Drawing for the job (mm, zero at the part's lowest x, y, z). Round coordinates to 2 decimals unless told otherwise and drop trailing zeros. Write each loop counter-clockwise with the first axis right and the second up, starting at its lowest first coordinate (ties: lowest second). Pieces come first, ordered by that corner, then holes. Notation, with made-up numbers: (-23.75, 77.25) - (3.25, 77.25) arc R21 cw to (3.25, 106.25) - close; hole circle Ø5 at (-19.75, 24). An arc over 180 degrees is marked (long way). One line per question, with ' | ' between items.
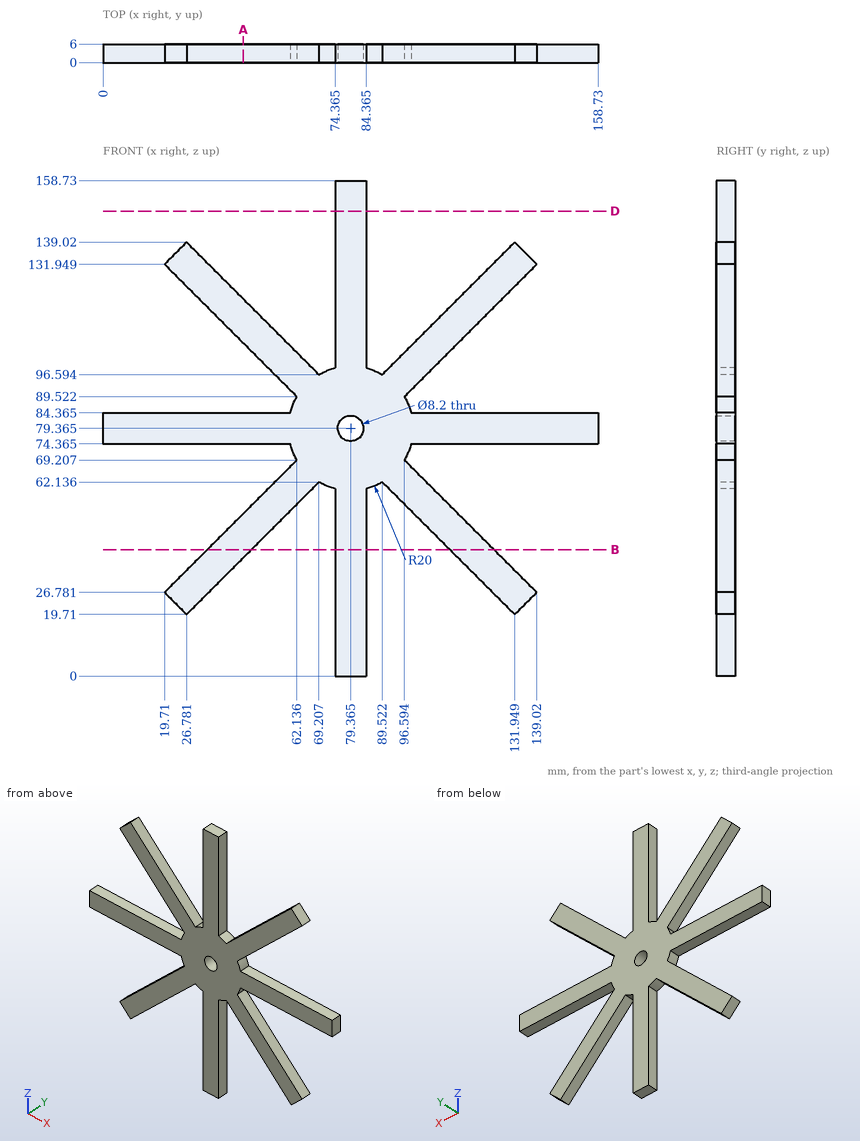
Q1. Drop flat-ended pins along their axis: pin 1 (1 mm diameter, centred on y = 2, z = 16, fed in from -X) (1 decimal); pin 2 (1.5 mm diameter, centred on x = 114.5, y = 3.5, fed in from +Z); pin 3 (3 mm diameter, centred on x = 19, y = 2.5, fed in from +Z); pin 4 (1 mm diameter, centred on x = 115.5, z = 107.5, fed in from +Y). Give the stop position or say it passes through.
Found:
pin 1: x = 74.4 | pin 2: z = 122.32 | pin 3: z = 132.74 | pin 4: through
Q2. Saw through at B-B, the plane z = 40.5. List the corners of the cut face in (x, y) (1 decimal).
Found:
outline: (33.4, 0) - (47.6, 0) - (47.6, 6) - (33.4, 6) - close; (74.4, 0) - (84.4, 0) - (84.4, 6) - (74.4, 6) - close; (111.2, 0) - (125.3, 0) - (125.3, 6) - (111.2, 6) - close
Q3. Drill centre lines: L1, parallel to Z at x = 112.5, y = 0.85 (1 decimal); L2, parallel to X at y = 2.9, z = 57.5 (1 decimal); L3, parallel to X at y = 0.8, z = 41.5 (1 decimal). Where is each one in solid material? Low to high. Write a range as from..to.
Found:
L1: 39.2..53.3, 74.4..84.4, 105.4..119.6 | L2: 50.4..64.6, 74.4..84.4, 94.2..108.3 | L3: 34.4..48.6, 74.4..84.4, 110.2..124.3
Q4. Saw through at A-A, the plane x = 45. List the corners of the cut face in (y, z) (1 decimal), then the cut area to 3 significant figures.
Found:
outline: (0, 37.9) - (6, 37.9) - (6, 52.1) - (0, 52.1) - close; (0, 74.4) - (6, 74.4) - (6, 84.4) - (0, 84.4) - close; (0, 106.7) - (6, 106.7) - (6, 120.8) - (0, 120.8) - close | area: 230 mm^2
Q5. Saw through at D-D, the plane z = 149. List the corners of the cut face in (x, y) (1 decimal).
Found:
outline: (74.4, 0) - (84.4, 0) - (84.4, 6) - (74.4, 6) - close
